Autodesk Inventor part; units mm, degrees
ref_plane "Work Plane1" through (-48.366, 22.225, 28.1991) normal (0, 0, 1) x (1, 0, 0)
ref_plane "YZ Plane" through (0, 0, 0) normal (1, 0, 0) x (0, 1, 0)
ref_plane "XZ Plane" through (0, 0, 0) normal (0, 1, 0) x (-1, 0, 0)
sketch "Sketch1" plane through (0, 0, 0) normal (0, 0, 1) x (1, 0, 0)
  circle A0 centre (12.2387, 16.51) radius 2.54
  line L0 (19.8587, 0) -> (0, 0)
  line L1 (19.8587, 0) -> (19.8587, 22.225)
  line L2 (0, 22.225) -> (19.8587, 22.225)
  line L3 (0, 0) -> (0, 22.225)
  line L4 (-42.016, 22.225) -> (-42.016, 0)
  line L5 (-42.016, 22.225) -> (19.8587, 22.225)
  line L6 (19.8587, 22.225) -> (19.8587, 0)
  line L7 (19.8587, 0) -> (-42.016, 0)
  line L8 (-42.016, 0) -> (-42.016, 22.225)
ref_plane "Work Plane1" through (-48.366, 22.225, 28.1991) normal (0, 0, 1) x (1, 0, 0)
extrude "Extrusion1" add sketch "Sketch1" along normal up to surface (28.1991 mm away) contours A0 | L0 L3 L2 L1 | L7 L4 L5 L3
sketch "Sketch6" plane through (-42.016, 22.225, 0) normal (0, 1, 0) x (1, 0, 0)
  arc A0 (36.4747, -28.1991) -> (61.8747, -2.7991) centre (36.4747, -2.7991) ccw
  arc A1 (-11.8913, 0) -> (42.016, 0) centre (15.0623, 38.2739) ccw
  line L0 (0, -17.4041) -> (38.1, -17.4041)
  line L1 (0, 0) -> (0, -28.1991)
  line L2 (0, -6.049) -> (0, 0)
  line L3 (0, 0) -> (42.016, 0)
  line L4 (61.8747, 0) -> (61.8747, -28.1991)
  line L5 (61.8747, -2.7991) -> (61.8747, -28.1991)
  line L6 (61.8747, -28.1991) -> (36.4747, -28.1991)
  line L7 (38.1, -17.4041) -> (38.1, -28.147)
  line L8 (0, -17.4041) -> (0, -6.049)
  line L9 (61.8747, -28.1991) -> (0, -28.1991)
  line L10 (38.1, -28.1991) -> (36.4747, -28.1991)
  line L11 (38.1, -17.4041) -> (0, -17.4041)
  line L12 (0, -17.4041) -> (0, -28.1991)
  line L13 (0, -28.1991) -> (38.1, -28.1991)
  line L14 (38.1, -28.1991) -> (38.1, -17.4041)
  line L15 (0, -23.7541) -> (38.1, -23.7541)
  line L16 (0, -28.1991) -> (38.9215, -28.2018)
  line L17 (38.9215, -28.2018) -> (38.9212, -28.1991)
  line L18 (36.4747, -20.5791) -> (38.1, -20.5791)
  line L19 (36.4747, -20.5791) -> (0, -20.5791)
extrude "Extrusion6" cut sketch "Sketch6" against normal through all contours L9 L1 L15 L7 A0 | A0 L14 L6 | L6 L17 L16 L9 | L1 L3 A1 | A0 L4 L6 L14 | L15 L1 L19 L18 L7
sketch "Sketch7" plane through (-42.016, 0, 6.049) normal (-1, 0, 0) x (0, 0, 1)
  line L0 (16.1176, 18.669) -> (12.9426, 18.669)
  circle A0 centre (14.5301, 10.922) radius 3.175
  arc A1 (12.8156, 13.744) -> (16.2446, 13.744) centre (14.5301, 10.922) ccw
  line L1 (16.2446, 18.796) -> (16.2446, 10.795)
  line L2 (16.2446, 10.795) -> (12.8156, 10.795)
  line L3 (12.8156, 10.795) -> (12.8156, 18.796)
  line L4 (12.8156, 17.399) -> (16.2446, 17.399)
  point P0 (-6.049, 0)
  dimension "d31" = 6.604
  dimension "d35" = 6.477
extrude "Extrusion7" cut sketch "Sketch7" against normal blind 38.1
sketch "Sketch8" plane through (-42.016, 0, 20.5791) normal (0, 0, 1) x (1, 0, 0)
  line L0 (0, 14.097) -> (33.655, 14.097)
  line L1 (38.1, 7.62) -> (0, 7.62)
  line L2 (0, 14.097) -> (0, 7.62)
  line L3 (0, 13.744) -> (38.1, 13.744)
  line L4 (0, 22.225) -> (0, 0)
  line L5 (38.1, 10.8585) -> (0, 10.8585)
  line L6 (9.525, 13.6716) -> (5.08, 13.6716)
  line L7 (9.525, 13.6716) -> (9.525, 17.272)
  line L8 (9.525, 17.272) -> (5.08, 17.272)
  line L9 (5.08, 17.272) -> (5.08, 13.6716)
  line L10 (19.05, 13.6716) -> (14.605, 13.6716)
  line L11 (19.05, 13.6716) -> (19.05, 17.272)
  line L12 (19.05, 17.272) -> (14.605, 17.272)
  line L13 (14.605, 17.272) -> (14.605, 13.6716)
  line L14 (28.575, 13.6716) -> (24.13, 13.6716)
  line L15 (28.575, 13.6716) -> (28.575, 17.272)
  line L16 (28.575, 17.272) -> (24.13, 17.272)
  line L17 (24.13, 17.272) -> (24.13, 13.6716)
  line L18 (38.1, 13.6716) -> (33.655, 13.6716)
  line L19 (38.1, 13.6716) -> (38.1, 17.272)
  line L20 (38.1, 17.272) -> (33.655, 17.272)
  line L21 (33.655, 17.272) -> (33.655, 13.6716)
  line L22 (0, 10.8585) -> (5.08, 10.8585)
  line L23 (5.08, 10.8585) -> (5.08, 19.7485)
  line L24 (5.08, 19.7485) -> (0, 19.7485)
  line L25 (0, 19.7485) -> (0, 10.8585)
  line L26 (9.525, 10.8585) -> (14.605, 10.8585)
  line L27 (14.605, 10.8585) -> (14.605, 19.7485)
  line L28 (14.605, 19.7485) -> (9.525, 19.7485)
  line L29 (9.525, 19.7485) -> (9.525, 10.8585)
  line L30 (19.05, 19.7485) -> (24.13, 19.7485)
  line L31 (24.13, 19.7485) -> (24.13, 10.8585)
  line L32 (24.13, 10.8585) -> (19.05, 10.8585)
  line L33 (19.05, 10.8585) -> (19.05, 19.7485)
  line L34 (28.575, 10.8585) -> (33.655, 10.8585)
  line L35 (33.655, 10.8585) -> (33.655, 19.7485)
  line L36 (33.655, 19.7485) -> (28.575, 19.7485)
  line L37 (28.575, 19.7485) -> (28.575, 10.8585)
  point P0 (42.016, 0)
  dimension "d36" = 8.89
revolve "Revolution2" cut sketch "Sketch8" angle 360 about axis through (-3.916, 10.8585, 20.5791) along (-1, 0, 0) contours L4 L24 L23 L9 L0 | L0 L9 L3 L2 | L3 L9 L23 L5 L2 | L7 L29 L28 L27 L13 L0 | L0 L13 L3 L7 | L3 L13 L27 L5 L29 L7 | L11 L33 L30 L31 L17 L0 | L0 L17 L3 L11 | L3 L17 L31 L5 L33 L11 | L15 L37 L36 L35 L21 L0 | L0 L21 L3 L15 | L3 L21 L35 L5 L37 L15
sketch "Sketch9" plane through (-42.016, 22.225, 20.5791) normal (0, 0, 1) x (1, 0, 0)
  line L0 (19.05, -4.826) -> (19.05, -2.4765)
  line L1 (19.05, -2.4765) -> (24.13, -2.4765)
  line L2 (24.13, -2.4765) -> (24.13, -4.826)
  line L3 (24.13, -4.826) -> (28.575, -4.826)
  line L4 (28.575, -4.826) -> (28.575, -2.4765)
  line L5 (28.575, -2.4765) -> (33.655, -2.4765)
  line L6 (33.655, -2.4765) -> (33.655, -4.826)
  line L7 (33.655, -4.826) -> (38.1, -4.826)
  line L8 (38.1, 0) -> (38.1, -4.826)
  line L9 (0, 0) -> (38.1, 0)
  line L10 (0, -2.4765) -> (0, 0)
  line L11 (0, -2.4765) -> (5.08, -2.4765)
  line L12 (5.08, -2.4765) -> (5.08, -4.826)
  line L13 (5.08, -4.826) -> (9.525, -4.826)
  line L14 (9.525, -4.826) -> (9.525, -2.4765)
  line L15 (9.525, -2.4765) -> (14.605, -2.4765)
  line L16 (14.605, -2.4765) -> (14.605, -4.826)
  line L17 (14.605, -4.826) -> (19.05, -4.826)
  circle A0 centre (7.3025, -2.4765) radius 1.27
  line L18 (19.05, -20.2565) -> (19.05, -14.605)
  line L19 (19.05, -14.605) -> (14.605, -14.605)
  line L20 (14.605, -14.605) -> (14.605, -20.2565)
  line L21 (14.605, -20.2565) -> (9.525, -20.2565)
  line L22 (9.525, -20.2565) -> (9.525, -14.605)
  line L23 (9.525, -14.605) -> (5.08, -14.605)
  line L24 (5.08, -14.605) -> (5.08, -20.2565)
  line L25 (5.08, -20.2565) -> (0, -20.2565)
  line L26 (0, -22.225) -> (0, -20.2565)
  line L27 (38.1, -22.225) -> (0, -22.225)
  line L28 (38.1, -14.605) -> (38.1, -22.225)
  line L29 (38.1, -14.605) -> (33.655, -14.605)
  line L30 (33.655, -14.605) -> (33.655, -20.2565)
  line L31 (33.655, -20.2565) -> (28.575, -20.2565)
  line L32 (28.575, -20.2565) -> (28.575, -14.605)
  line L33 (28.575, -14.605) -> (24.13, -14.605)
  line L34 (24.13, -14.605) -> (24.13, -20.2565)
  line L35 (24.13, -20.2565) -> (19.05, -20.2565)
  circle A1 centre (35.8775, -20.2565) radius 1.27
  circle A2 centre (35.8775, -2.4765) radius 1.27
  circle A3 centre (7.3025, -20.2565) radius 1.27
  point P0 (42.016, -22.225)
  dimension "d38" = 2.54
  dimension "d39" = 2.54
  dimension "d40" = 2.54
  dimension "d41" = 2.54
extrude "Extrusion8" cut sketch "Sketch9" against normal blind 6.35 contours A0 | A1 | A2 | A3
sketch "Sketch10" plane through (0, 22.225, 0) normal (0, 1, 0) x (1, 0, 0)
  arc A0 (-42.016, -6.049) -> (0, 0) centre (-26.9537, 38.2739) ccw
  line L0 (-42.016, -6.049) -> (-42.016, -20.5791)
  line L1 (-42.016, -20.5791) -> (-3.916, -20.5791)
  line L2 (-3.916, -20.5791) -> (-3.916, -28.147)
  arc A1 (-3.916, -28.147) -> (19.8587, -2.7991) centre (-5.5413, -2.7991) ccw
  line L3 (19.8587, 0) -> (19.8587, -2.7991)
  line L4 (19.8587, 0) -> (0, 0)
  line L5 (0, 0) -> (19.8587, 0)
  arc A2 (-45.191, -4.8398) -> (0, 0) centre (-26.9537, 38.2739) ccw
  line L6 (-42.016, -20.5791) -> (-45.191, -20.5791)
  line L7 (-45.191, -20.5791) -> (-45.191, -4.8398)
  line L8 (-42.016, -6.049) -> (-42.016, -20.5791)
extrude "Extrusion9" add sketch "Sketch10" against normal up to surface (22.225 mm away) contours L0 L6 L7 A2
sketch "Sketch11" plane through (-36.936, 1.9685, 20.5791) normal (-1, 0, 0) x (0, 0, 1)
  line L0 (-1.7145, 15.4305) -> (0, 15.4305)
  line L1 (0, 19.05) -> (0, 16.51)
  line L2 (0, 20.2565) -> (0, 15.4305)
  line L3 (7.5679, 20.2565) -> (-17.78, 20.2565)
  line L4 (-1.7145, 11.7755) -> (-1.7145, 15.4305)
  arc A0 (-1.7145, 11.7755) -> (0, 5.6515) centre (0, 8.9535) ccw
  line L5 (0, 0) -> (0, 5.6515)
  line L6 (0, 1.27) -> (0, -1.27)
  line L7 (0, 5.6515) -> (0, -1.9685)
  arc A1 (0, 17.78) -> (0, 0) centre (0, 8.89) ccw
  line L8 (-1.7145, 15.4305) -> (0, 15.4305)
  line L9 (0, 15.4305) -> (0, 5.6515)
  point P0 (-20.5791, -1.9685)
extrude "Extrusion10" cut sketch "Sketch11" along normal through all contours L0 L9 A0 L4
sketch "Sketch12" plane through (0, 0, 0) normal (0, 0, -1) x (-1, 0, 0)
  circle A0 centre (-12.2387, 16.51) radius 2.54
  circle A1 centre (-12.2387, 16.51) radius 2.54
  line L0 (0.9001, 2.794) -> (-17.0647, 2.794)
  line L1 (0.9001, 2.794) -> (0.9001, 22.225)
  line L2 (-17.0647, 22.225) -> (0.9001, 22.225)
  line L3 (-17.0647, 2.794) -> (-17.0647, 22.225)
  line L4 (60.812, 2.794) -> (60.812, 18.669)
  line L5 (60.812, 18.669) -> (51.9355, 18.669)
  line L6 (51.9355, 18.669) -> (51.9355, 2.794)
  line L7 (70.972, 2.794) -> (60.812, 2.794)
  line L8 (-17.0647, 2.794) -> (-6.9047, 2.794)
  line L9 (-6.9047, 2.794) -> (-6.9047, 19.939)
  line L10 (-6.9047, 19.939) -> (-17.0647, 19.939)
  line L11 (-17.0647, 19.939) -> (-17.0647, 2.794)
  line L12 (3.916, 0) -> (3.916, 22.225)
  point P0 (0, 0)
revolve "Revolution3" cut sketch "Sketch12" angle 80 about axis through (-3.916, 0, 0) along (0, -1, 0) contours A0 | L0 L3 L10 L9
sketch "Sketch13" plane through (6.9047, 19.939, 0) normal (0, -1, 0) x (1, 0, 0)
  arc A0 (10.16, 0) -> (-7.1774, 20.6619) centre (-10.8207, 0) ccw
  line L0 (-8.9417, 10.6563) -> (-7.1774, 20.6619)
  arc A1 (0, 0) -> (-8.9417, 10.6563) centre (-10.8207, 0) ccw
  arc A2 (-2.5072, 15.3858) -> (-4.0166, 12.5925) centre (-3.2619, 13.9892) ccw
  arc A3 (-5.6768, 9.5199) -> (-8.9417, 10.6563) centre (-10.8207, 0) ccw
  arc A4 (-0.847, 18.4585) -> (-7.1774, 20.6619) centre (-10.8207, 0) ccw
  line L1 (-7.1774, 20.6619) -> (-8.9417, 10.6563)
  arc A5 (-0.847, 18.4585) -> (-8.0596, 15.6591) centre (-3.2619, 13.9892) ccw
  arc A6 (-8.3414, 14.0608) -> (-5.6768, 9.5199) centre (-3.2619, 13.9892) ccw
  arc A7 (-0.847, 18.4585) -> (-8.0596, 15.6591) centre (-3.2619, 13.9892) ccw
  arc A8 (-8.3414, 14.0608) -> (-5.6768, 9.5199) centre (-3.2619, 13.9892) ccw
  arc A9 (6.6675, 0) -> (-2.5072, 15.3858) centre (-10.8207, 0) ccw
  arc A10 (3.4925, 0) -> (-4.0166, 12.5925) centre (-10.8207, 0) ccw
  line L2 (6.6675, 0) -> (3.4925, 0)
  line L3 (-6.9047, 0) -> (12.954, 0)
  dimension "d52" = 3.175
extrude "Extrusion11" add sketch "Sketch13" along normal up to next contours A5 L0 A0 | L2 A10 A2 A9 | A6 A1 L0
chamfer "Chamfer1" [suppressed]
fillet "Fillet1" [suppressed]
fillet "Fillet2" [suppressed]
properties part number "final lock housing back"
For this review, take the finished solid that the model builds, in its own axes (mm). A direction names the side the tool comes from. Give positions to 0.01 mm unless a question says otherwise; leave off trailing zeros. Order: outer loops, then holes, each group sorted by start corner. A loop starts at its lowest first (then second) coordinate and runs counter-clockwise, first axis right, second up.
1) Insertion check: pin 1 (3.5 mm diameter, centred on x = -44.5, y = 16, fed in from +Z); pin 2 (9.5 mm diameter, centred on x = 6.5, z = 12.5, fed in from -Y); pin 3 (1.5 mm diameter, centred on x = -34.71, y = 1.97, fed in from -Z); pin 4 (4.5 mm diameter, centred on y = 7.5, z = 17.5, fed in from +X). Each pin has a flat end and moves straight along its axis. Give the tip position at first contact, or say it passes through.
2) The part is to be moulded in two halves that separate along Y. For faces 5 (the face through (-12, 0, 14)), 6 (the face through (-24, 4, 20.579)), 7 (the face through (-44, 16, 18.865)), 8 (the face through (-20.39, 10.66, 11.69)), say which applies: released by +Y, released by -Y, zero draft, split by the parting line, or undercut.
3) Take a section at C-C (x = 5). Give the boundary of the cut face in (y, z) (3 decimals).
4) Take a section at B-B (z = 4). Give the boundary of the cut face in (x, y) (3 decimals).
5) Take a section at D-D (x = 12). Give the boundary of the cut face in (y, z) (3 decimals).
6) Wall thickness on line 1 (Y direction, x = 16, z = 1.5) (3 decimals); line 2 (X direction, y = 20.5, z = 16.75); line 3 (X direction, y = 8, z = 10.25): over which ranges is each line inside the solid? List them lowest first.
7) For faces 1 (the face through (14.023, 11.487, 10.881)), 2 (the face through (-6, 20, 14.229)), 3 (the face through (12.8, 11.27, 20.37)), 4 (the face through (-6, 17.399, 20)), list the 3-axis set-ups (+Z, -Z, +X, -X, +Y, -Y) from which the entire face can be reached by the end or side of a thin tool; tool diameter is ignored.
Derived:
1. pin 1: stops at z = 20.58
1. pin 2: stops at y = 0
1. pin 3: stops at z = 7.76
1. pin 4: stops at x = 16.6
2. face 5: released by -Y
2. face 6: zero draft
2. face 7: undercut
2. face 8: undercut
3. outline: (0, 0) - (22.225, 0) - (22.225, 25.908) - (0, 25.908) - close; hole (2.794, 6.131) - (19.939, 6.131) - (19.939, 11.197) - (2.794, 11.197) - close; hole (2.794, 15.045) - (19.939, 15.045) - (19.939, 18.885) - (2.794, 18.885) - close
4. outline: (-6.846, 0) - (19.83, 0) - (19.83, 22.225) - (-6.846, 22.225) - close; hole (6.138, 2.794) - (9.827, 2.794) - (9.827, 19.939) - (6.138, 19.939) - close; hole (13.109, 2.794) - (16.68, 2.794) - (16.68, 19.939) - (13.109, 19.939) - close
5. outline: (0, 0) - (22.225, 0) - (22.225, 21.169) - (0, 21.169) - close; hole (2.794, 7.247) - (19.939, 7.247) - (19.939, 13.67) - (2.794, 13.67) - close
6. line 1: y = 0 to 2.794, 19.939 to 22.225
6. line 2: x = -45.19 to -35.74, -33.69 to -7.16, -5.11 to 15.68
6. line 3: x = -45.19 to 0.2, 6.07 to 10.25, 14.39 to 18.74
7. face 1: none
7. face 2: +Z
7. face 3: +Z, +X, +Y, -Y
7. face 4: +Z, -X
